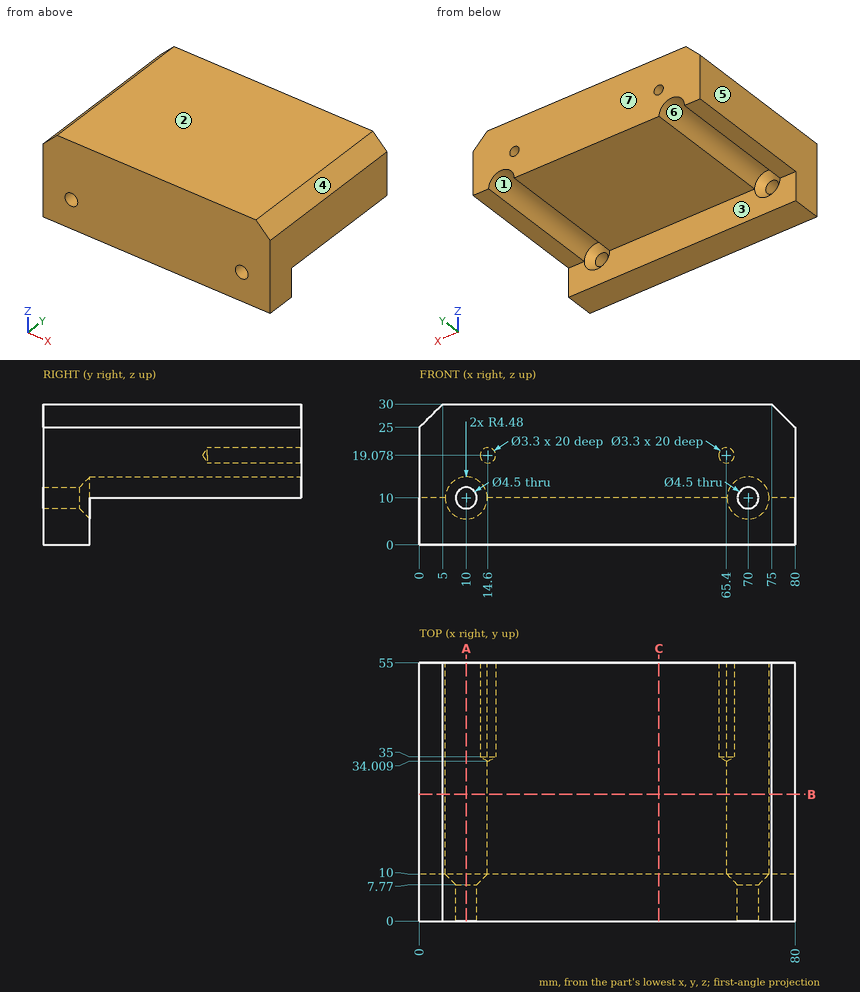
Input: dimensioned drawing with shaded views. Units: mm. Origin: part minimum x, y, z. A direction names the side the tool comes from. Coordinates: 2 decimals unless noted, no trailing zeros. Loops run counter-clockwise (first coordinate to the right, second up) from the corner with the lowest first, then second, coordinate; pieces in that order, holes last. Notation, with made-up numbers: M -30,-37.75 L -16,-37.75 A21 cw -16,-9.75 Z; hole C -17,-9.5 d4. An arc over 180 degrees is marked long. Put each result on its own line as item: value.
(1) Access query for the marked faces 1, 2 and 3. Directions: +Z, -Z, +X, -X, +Y, -Y. A direction counts if a zero-diameter tool reaches every point of the face in a straight line with its end or side. Return the directions, or none.
Answer sheet:
face 1: -Z, +Y
face 2: +Z, +X, -X, +Y, -Y
face 3: -Z, +X, -X, +Y
(2) Cut plane B-B on y = 27. Return the cut outline in (x, z).
Answer sheet:
outline: M 0,10 L 5.52,10 A4.48 cw 14.48,10 L 65.52,10 A4.48 cw 74.48,10 L 80,10 L 80,25 L 75,30 L 5,30 L 0,25 Z
(3) Draft query along X for the marked faces 4, 5, 6 and 7. Return one class per face: pulls with the +X half, pulls with the -X half, needs draft (parallel to the pull), parting line crosses it, or undercut.
Answer sheet:
face 4: pulls with the +X half
face 5: pulls with the -X half
face 6: undercut
face 7: needs draft
(4) Cut plane C-C on x = 51. Return the cut outline in (y, z), then the cut area to 3 significant figures.
Answer sheet:
outline: M 0,0 L 10,0 L 10,10 L 55,10 L 55,30 L 0,30 Z
area: 1,200 mm^2
(5) First-contact query: pin 1 (6 mm diameter, centred on x = 20.5, y = 20.5, fed in from -Z); pin 2 (3 mm diameter, centred on x = 48, z = 4.5, fed in from +Y); pin 3 (6 mm diameter, centred on x = 10, z = 10, fed in from +Y). Flat tips, straight axial feed; report the tip coordinate or a pass-through.
Answer sheet:
pin 1: stops at z = 10
pin 2: stops at y = 10
pin 3: stops at y = 8.52
(6) Material intervals for probe 1 along X at (y, z) = (3.75, 10); probe 2 along X at (y, z) = (37.5, 19.25); probe 3 along Z at (x, y) = (10, 4), sorted ascending.
Answer sheet:
probe 1: x = 0 to 7.75, 12.25 to 67.75, 72.25 to 80
probe 2: x = 0 to 12.96, 16.24 to 63.76, 67.04 to 80
probe 3: z = 0 to 7.75, 12.25 to 30
(7) Cut plane A-A on x = 10. Return the cut outline in (y, z).
Answer sheet:
outline: M 0,0 L 10,0 L 10,5.52 L 7.77,7.75 L 0,7.75 Z; M 0,12.25 L 7.77,12.25 L 10,14.48 L 55,14.48 L 55,30 L 0,30 Z
